The listing builds one solid part. Answer for the finished solid, in the listing's coordinates (mm). A direction names the side the tool comes from. Coordinates: 2 decimals unless noted, no trailing zeros. Order: outer loops, then holes, each group sorted by start corner. A loop starts at its lowest first (then second) coordinate and runs counter-clockwise, first axis right, second up. Notation, with made-up numbers: M 16,-27 L 50,-27 A17 ccw 50,-16 Z; hole C -24.5,74 d3. An arc over 180 degrees is marked long. One line per item, written item: value. Start each with the question number.
Q1. Determine the mould class of faces 1 (the flat face through (-3, 12, 40)), 2 (the cylindrical face through (-0.065, 15.496, 19.72)), 3 (the cylindrical face through (0, 12, 20)), 4 (the cylindrical face through (9.84, -8.78, 38.72)) for opening direction Y: pulls with the +Y half, pulls with the -Y half, needs draft (parallel to the pull), parting line crosses it, or undercut.
Q2. Straight lines are drawn through the part: line 1 along Y through (x, z) = (0, 32.5); line 2 along X through (y, z) = (-6, 38); line 3 along Y through (x, z) = (5.75, 8). For each, find the intervals that lie inside material, in ascending order. Write a range as [from, to].
Q3. The part is cut by section D-D on y = -2. Give the vertices of the cut face in (x, z), then the cut area to 3 significant figures.
Q4. The part is cut by section B-B on x = 0. Give the vertices of the cut face in (y, z).
Q5. For faces 5 (the flat face through (3, 14, 20)), 6 (the flat face through (-3, 12, 0)), 7 (the flat face through (9.5, -8, 39)), determine the directions among +Z, -Z, +X, -X, +Y, -Y from which every point of the face is accessible in a straight line to the end or side of a thin tool.
Q6. The part is cut by section C-C on z = 31. Give the vertices of the cut face in (x, y), then the cut area to 3 significant figures.
Q7. The part is cut by section A-A on y = 10. Give the vertices of the cut face in (x, z), then the cut area to 3 significant figures.
Q8. Each of these flat-tipped pins is pushed along its axis until it touches: pin 1 Ø2 at (y, z) = (14.5, 15) entering from -X; pin 2 Ø5 at (x, z) = (7, 29.5) entering from +Y; pin 3 Ø1.1 at (y, z) = (-7.5, 39) entering from -X. Where does it stop, or does it pass through?
```python
from build123d import *

# Parameters (mm, degrees)
F1_DEPTH    = 40
F2_R        = 17.5
F3_DEPTH    = 15
F5_R        = 0.5
F6_DEPTH    = 40
F7_T1_DEPTH = 9.1201245228
F7_T3_DEPTH = 9.1201245228


# Not quite as in the source:
# - a fillet or chamfer that OpenCascade refuses, or shapes differently, is made with other operations: its cross-section is extruded or revolved along the edge and cut away or added


with BuildPart() as f1:
    # F0 (on Top) → F1 (new body)
    with BuildSketch(Plane.XY):
        with BuildLine():
            ThreePointArc((-9.5, -7.3314391493), (0, 12), (9.5, -7.3314391493))
            Line((9.5, -7.3314391493), (9.5, -9.5916630466))
            ThreePointArc((9.5, -9.5916630466), (0, 13.5), (-9.5, -9.5916630466))
            Line((-9.5, -9.5916630466), (-9.5, -7.3314391493))
        make_face()
    extrude(amount=F1_DEPTH)


with BuildPart() as f3:
    # F2 (on Right) → F3 (new body, symmetric)
    with BuildSketch(Plane.YZ):
        with Locations((-8, 20)):
            Circle(F2_R)
    extrude(amount=F3_DEPTH, both=True)


with BuildPart() as f1_1:
    add(f1.part)

    # F4: cut F3
    add(f3.part, mode=Mode.SUBTRACT)

    # F5 (on Top) → F6 (join)
    with BuildSketch(Plane.XY):
        with BuildLine():
            Line((2.9997656158, 13.1625), (2.9997656158, 14.9625))
            ThreePointArc((2.9997656158, 14.9625), (0, 18), (-2.9997656158, 14.9625))
            Line((-2.9997656158, 14.9625), (-2.9997656158, 13.1625))
            ThreePointArc((-2.9997656158, 13.1625), (0, 13.5), (2.9997656158, 13.1625))
        make_face()
        with Locations((0, 15)):
            Circle(F5_R, mode=Mode.SUBTRACT)
    extrude(amount=F6_DEPTH)

    # F7: fillet of radius 0.5 on 4 edges, made by hand

    # F7_s2 → F7_t1 (cut)
    with BuildSketch(Plane.XY.offset(34.1536712775)):
        with BuildLine():
            ThreePointArc((-10.3846153846, -8.6261093961), (-9.8301584449, -8.7768938345), (-9.5, -8.3066238629))
            Line((-9.5, -8.3066238629), (-9.5, -9.5916630466))
            ThreePointArc((-9.5, -9.5916630466), (-9.9540220872, -9.1196186482), (-10.3846153846, -8.6261093961))
        make_face()
        with BuildLine():
            ThreePointArc((10.3846153846, -8.6261093961), (9.8301584449, -8.7768938345), (9.5, -8.3066238629))
            Line((9.5, -8.3066238629), (9.5, -9.5916630466))
            ThreePointArc((9.5, -9.5916630466), (9.9540220872, -9.1196186482), (10.3846153846, -8.6261093961))
        make_face()
    extrude(amount=F7_T1_DEPTH, mode=Mode.SUBTRACT)

    # F7_s4 → F7_t3 (cut)
    with BuildSketch(Plane.XY.offset(-3.2737958003)):
        with BuildLine():
            ThreePointArc((9.5, -8.3066238629), (9.8301584449, -8.7768938345), (10.3846153846, -8.6261093961))
            ThreePointArc((10.3846153846, -8.6261093961), (9.9540220872, -9.1196186482), (9.5, -9.5916630466))
            Line((9.5, -9.5916630466), (9.5, -8.3066238629))
        make_face()
        with BuildLine():
            ThreePointArc((-9.5, -8.3066238629), (-9.8301584449, -8.7768938345), (-10.3846153846, -8.6261093961))
            ThreePointArc((-10.3846153846, -8.6261093961), (-9.9540220872, -9.1196186482), (-9.5, -9.5916630466))
            Line((-9.5, -9.5916630466), (-9.5, -8.3066238629))
        make_face()
    extrude(amount=F7_T3_DEPTH, mode=Mode.SUBTRACT)


solid = f1_1.part
```
Output:
1. face 1: needs draft
1. face 2: undercut
1. face 3: undercut
1. face 4: pulls with the -Y half
2. line 1: y = [12, 14.5], [15.5, 18]
2. line 2: x = [-12.09, -10.39], [10.39, 12.09]
2. line 3: y = [10.53, 12.21]
3. outline: M -13.35,0 L -11.83,0 L -11.83,3.56 L -13.35,3.56 Z; M -13.35,36.44 L -11.83,36.44 L -11.83,40 L -13.35,40 Z; M 11.83,0 L 13.35,0 L 13.35,3.56 L 11.83,3.56 Z; M 11.83,36.44 L 13.35,36.44 L 13.35,40 L 11.83,40 Z
3. area: 21.6 mm^2
4. outline: M 12,0 L 14.5,0 L 14.5,40 L 12,40 Z; M 15.5,0 L 18,0 L 18,40 L 15.5,40 Z
5. face 5: +Z, -Z, +X, +Y
5. face 6: -Z, +X, -X, +Y, -Y
5. face 7: +Z, -Z, -Y
6. outline: M -12.28,5.61 L -10.61,5.61 A12 cw 10.61,5.61 L 12.28,5.61 A13.5 ccw 3,13.16 L 3,14.96 A3 ccw long -3,14.96 L -3,13.16 A13.5 ccw Z; hole C 0,15 d1
6. area: 65.7 mm^2
7. outline: M -9.07,0 L -6.63,0 L -6.63,40 L -9.07,40 Z; M 6.63,0 L 9.07,0 L 9.07,40 L 6.63,40 Z
7. area: 195 mm^2
8. pin 1: stops at x = -3
8. pin 2: stops at y = 12.73
8. pin 3: stops at x = -11.57
